```python
from build123d import *

# Parameters (mm, degrees)
F1_DEPTH = 80


# Not quite as in the source:
# - ends of sketch curves that miss each other by under 0.0002 mm in the source are joined


with BuildPart() as f1:
    # F0 (on Front) → F1 (new body)
    with BuildSketch(Plane.XZ):
        with BuildLine():
            Line((0, 20), (0, 0))
            Line((0, 0), (126.5, 0))
            Line((126.5, 0), (126.5, 5.872634))
            ThreePointArc((126.5, 5.872634), (126.4686827703, 5.9800868873), (126.3845387701, 6.0538885071))
            ThreePointArc((126.3845387701, 6.0538885071), (75.9297421053, 23.1880267358), (22.962901, 28.9999923785))
            ThreePointArc((22.962901, 28.9999923785), (22.9045566452, 28.9913078859), (22.8512831377, 28.9659817952))
            ThreePointArc((22.8512831377, 28.9659817952), (11.9447272771, 23.7801763601), (0, 22))
            Line((0, 22), (0, 20))
        make_face()
    extrude(amount=F1_DEPTH)


solid = f1.part
```
The listing builds one solid part. Answer for the finished solid, in the listing's coordinates (mm). Coordinates: 2 decimals unless noted, no trailing zeros. Write each loop counter-clockwise with the first axis right and the second up, starting at its lowest first coordinate (ties: lowest second). Pieces come first, ordered by that corner, then holes. Notation, with made-up numbers: (45, 37) -> (81, 37) arc R16 ccw to (81, 53) -> close; hole circle Ø3 at (52.25, -17). An arc over 180 degrees is marked (long way). Write each question's results on one line, items separated by ' | '. Start each with the question number.
1) A cutting plane is placed at C-C (x = 66). Determine the outline of the cut face in (y, z), then the cut area to 3 significant figures.
2) A cutting plane is placed at B-B (z = 23.75). Determine the outline of the cut face in (x, y).
3) Flat-ended cylindrical pins translate along their axes: pin 1 Ø10 at (x, y) = (62.5, -34) entering from +Z; pin 2 Ø1 at (y, z) = (-45, 10) entering from +X; pin 3 Ø2 at (y, z) = (-32.5, 7.5) entering from +X. Find the tip coordinate at first contact, or state that the pin passes through.
4) A cutting plane is placed at A-A (y = -59.5). Determine the outline of the cut face in (x, z).
5) Straight lines are drawn through the part: probe 1 along Z at (x, y) = (27.5, -17); probe 2 along Z at (x, y) = (59, -38); probe 3 along X at (y, z) = (-23.5, 6.75). For each, find the intervals that lie inside material, in ascending order.
Values follow:
1) outline: (-80, 0) -> (0, 0) -> (0, 25.18) -> (-80, 25.18) -> close | area: 2,010 mm²
2) outline: (11.85, -80) -> (73.33, -80) -> (73.33, 0) -> (11.85, 0) -> close
3) pin 1: z = 26.54 | pin 2: x = 118.65 | pin 3: x = 125.42
4) outline: (0, 0) -> (126.5, 0) -> (126.5, 5.87) arc R0.2 ccw to (126.38, 6.05) arc R244.82 ccw to (22.96, 29) arc R0.2 ccw to (22.85, 28.97) arc R40.96 cw to (0, 22) -> close
5) probe 1: 0 to 28.96 | probe 2: 0 to 26.32 | probe 3: 0 to 124.88
